Here's the drawing with two shaded views (mm, measured from the low corner). I have some questions. A direction names the side the tool comes from. Give positions to 0.01 mm unless a question says otherwise; leave off trailing zeros. Write each loop counter-clockwise with the first axis right and the second up, starting at its lowest first coordinate (ties: lowest second). Pieces come first, ordered by that corner, then holes. Notation, with made-up numbers: (-9, 83.5) -> (9, 83.5) arc R16 ccw to (9, 93.5) -> close; hole circle Ø6 at (-33.5, 10). An arc over 180 degrees is marked (long way). Put each result on its own line as item: value. Start each with the question number.
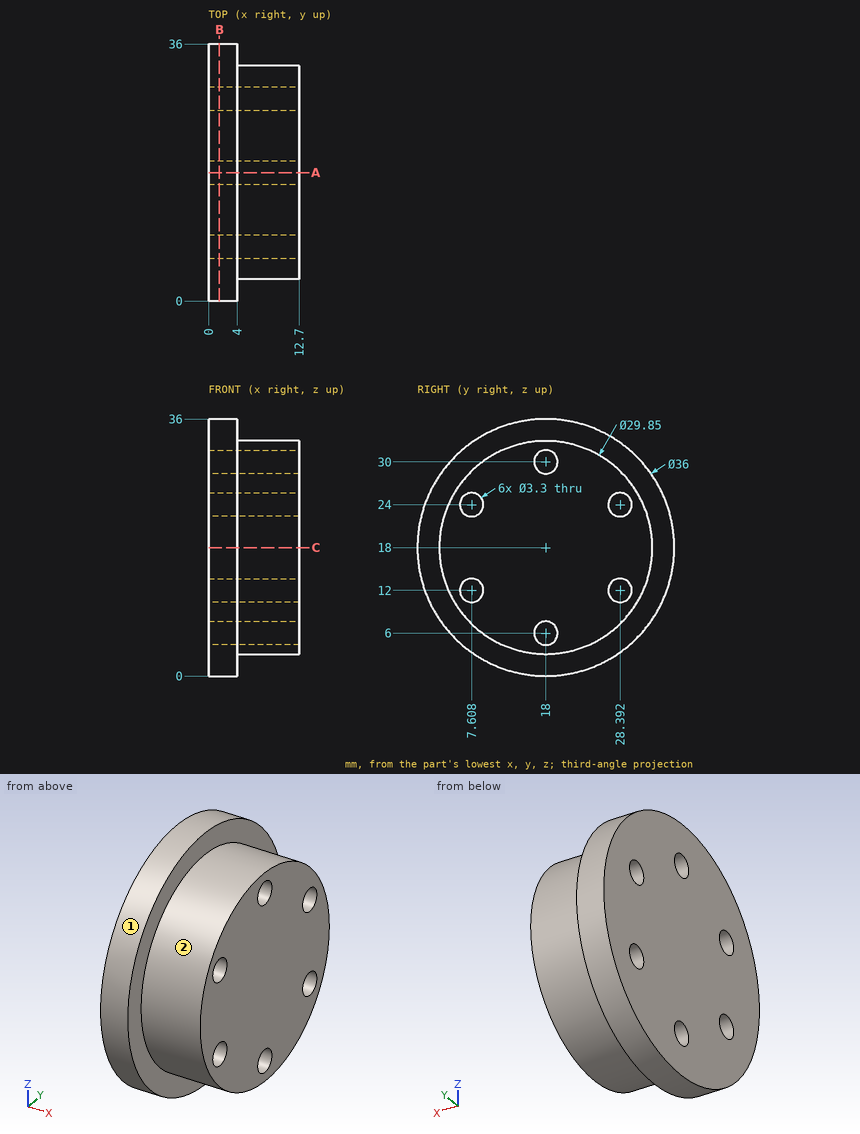
1) I need wall thicknesses on probe 1 along Y at (x, z) = (9.25, 13) (1 decimal); probe 2 along Z at (x, y) = (7, 28); probe 3 along Y at (x, z) = (3, 24). Which ranges of each line are inside material? Lowest first, please.
2) I'm going to push flat-ended pins straight in: pin 1 Ø3 at (x, y) = (3.5, 14.5) entering from +Z; pin 2 Ø6 at (x, z) = (11, 29) entering from +Y; pin 3 Ø2 at (y, z) = (18, 30) entering from +X; pin 4 Ø4 at (x, z) = (2, 28) entering from +Y (1 decimal). Where does each tip first touch, or does it pass through?
3) I want a section at C-C, the plane z = 18. Write out the boundary of the cut face in (x, y) (1 decimal), and give its area (3 significant figures).
4) Which directions (+Z, -Z, +X, -X, +Y, -Y) give clear straight access to the entire face, cutting with the end or side of a thin tool? Please do the marked faces 1 and 2.
5) I want a section at A-A, the plane y = 18. State how many separate pieces and enclosed holes the cut face has, and give its area (3 significant figures).
6) I want a section at B-B, the plane x = 1.5. Write out the boundary of the cut face in (y, z).
Established:
1. probe 1: y = 3.9 to 6.3, 8.9 to 27.1, 29.7 to 32.1
1. probe 2: z = 6.92 to 10.4, 13.6 to 22.4, 25.6 to 29.08
1. probe 3: y = 1.03 to 5.96, 9.26 to 26.74, 30.04 to 34.97
2. pin 1: stops at z = 35.89
2. pin 2: stops at y = 30.6
2. pin 3: passes through
2. pin 4: stops at y = 34.1
3. outline: (0, 0) -> (4, 0) -> (4, 3.1) -> (12.7, 3.1) -> (12.7, 32.9) -> (4, 32.9) -> (4, 36) -> (0, 36) -> close
3. area: 404 mm2
4. face 1: +X, -X
4. face 2: +X
5. separate pieces: 3
5. enclosed holes: 0
5. area: 320 mm2
6. outline: circle Ø36 at (18, 18); hole circle Ø3.3 at (7.61, 12); hole circle Ø3.3 at (7.61, 24); hole circle Ø3.3 at (18, 6); hole circle Ø3.3 at (18, 30); hole circle Ø3.3 at (28.39, 12); hole circle Ø3.3 at (28.39, 24)
